```python
from build123d import *

# Parameters (mm, degrees)
SKETCH1_W                                      = 120
SKETCH1_H                                      = 120
BOSS_EXTRUDE1_DEPTH                            = 3
SKETCH2_R                                      = 16
BOSS_EXTRUDE2_DEPTH                            = 8
BOSS_EXTRUDE2_DIRECTION_2_REACH                = 122.252
SKETCH3_R                                      = 13.75
CUT_EXTRUDE1_DEPTH                             = 122.407232036
CHAMFER1_SIZE                                  = 5
CSK_FOR_5_FLAT_HEAD_MACHINE_SCREW2_D           = 3.9116
CSK_FOR_5_FLAT_HEAD_MACHINE_SCREW2_DEPTH       = 10.1
CSK_FOR_5_FLAT_HEAD_MACHINE_SCREW2_CSINK_D     = 6.4008
CSK_FOR_5_FLAT_HEAD_MACHINE_SCREW2_CSINK_ANGLE = 82
CSK_FOR_5_FLAT_HEAD_MACHINE_SCREW2_TIP         = 1.175163199


with BuildPart() as part:
    # Sketch1 → Boss-Extrude1 (new body)
    with BuildSketch(Plane(origin=(0, 0, 0), x_dir=(1, 0, 0), z_dir=(0, 1, 0))):
        with Locations((0, -44)):
            Rectangle(SKETCH1_W, SKETCH1_H)
    extrude(amount=-BOSS_EXTRUDE1_DEPTH)

    # Sketch2 → Boss-Extrude2 (add)
    with BuildSketch(Plane(origin=(0, 1.389185421, -0.121537976), x_dir=(-1, 0, 0), z_dir=(0, 0.9961946980917455, -0.08715574274765836))):
        with Locations(Location((0, 0, 0), (0, 0, 90))):
            Circle(SKETCH2_R)
    extrude(amount=BOSS_EXTRUDE2_DEPTH)

    # Boss-Extrude2 direction 2: up to this face of the body (flat: up to its plane)
    boss_extrude2_direction_2_end = Plane(part.part.faces().sort_by_distance((0, 0, 44))[0])
    # Sketch2 → Boss-Extrude2 direction 2 (add, up to the picked face)
    with BuildSketch(Plane(origin=(0, 1.389185421, -0.121537976), x_dir=(-1, 0, 0), z_dir=(0, 0.9961946980917455, -0.08715574274765836)), mode=Mode.PRIVATE) as boss_extrude2_direction_2_sk1:
        with Locations(Location((0, 0, 0), (0, 0, 90))):
            Circle(SKETCH2_R)
    boss_extrude2_direction_2_tool1 = split(extrude(boss_extrude2_direction_2_sk1.sketch, amount=-BOSS_EXTRUDE2_DIRECTION_2_REACH, mode=Mode.PRIVATE), bisect_by=boss_extrude2_direction_2_end, keep=Keep.BOTH, mode=Mode.PRIVATE)
    add(boss_extrude2_direction_2_tool1.solids().sort_by(Axis((0, 1.389185, -0.121538), (0, -0.9961946980917455, 0.08715574274765836)))[0])

    # Sketch3 → Cut-Extrude1 (cut, through all)
    with BuildSketch(Plane(origin=(0, 9.358743006, -0.818783918), x_dir=(1, 0, 0), z_dir=(0, 0.9961946980917457, -0.08715574274765836))):
        with Locations(Location((0, 0, 0), (0, 0, 270))):
            Circle(SKETCH3_R)
    extrude(amount=-CUT_EXTRUDE1_DEPTH, mode=Mode.SUBTRACT)

    # Chamfer1
    # the kernel refuses this chamfer: 5 mm, written as the material it takes off along each edge
    with BuildSketch(Plane(origin=(60, 0, -28.85841494), x_dir=(-0.9996219169112968, 0.027495876610586372, 0), z_dir=(0, 0, 1)), Plane(origin=(72.85841494, 0, 104), x_dir=(0, 0.027495876610586334, -0.9996219169112968), z_dir=(-1, 0, 0)), Plane(origin=(-60, 0, 116.85841494), x_dir=(0.9996219169112968, 0.027495876610586372, 0), z_dir=(0, 0, -1))) as chamfer1_piece_1:
        Polygon((CHAMFER1_SIZE * 0.999621916911, CHAMFER1_SIZE * 0.0274958766106), (-CHAMFER1_SIZE * 0.0274958766106, CHAMFER1_SIZE * 0.999621916911), (0, 0), align=None)
    extrude(amount=145.71682988, mode=Mode.SUBTRACT)

    # CSK for #5 Flat Head Machine Screw2
    with Locations(Plane(origin=(0, 4.243645214, -16.432388249), x_dir=(0, -0.996194698092, 0.087155742748), z_dir=(0, -0.087155742748, -0.996194698092))):
        with Locations((0, 0)):
            CounterSinkHole(CSK_FOR_5_FLAT_HEAD_MACHINE_SCREW2_D / 2, CSK_FOR_5_FLAT_HEAD_MACHINE_SCREW2_CSINK_D / 2, depth=CSK_FOR_5_FLAT_HEAD_MACHINE_SCREW2_DEPTH, counter_sink_angle=CSK_FOR_5_FLAT_HEAD_MACHINE_SCREW2_CSINK_ANGLE)
            with Locations((0, 0, -(CSK_FOR_5_FLAT_HEAD_MACHINE_SCREW2_DEPTH + CSK_FOR_5_FLAT_HEAD_MACHINE_SCREW2_TIP / 2))):  # 118° drill point
                Cone(0, CSK_FOR_5_FLAT_HEAD_MACHINE_SCREW2_D / 2, CSK_FOR_5_FLAT_HEAD_MACHINE_SCREW2_TIP, mode=Mode.SUBTRACT)


solid = part.part
```
The listing builds one solid part. Answer for the finished solid, in the listing's coordinates (mm). Round coordinates to 2 decimals unless told otherwise and drop trailing zeros. Write each loop counter-clockwise with the first axis right and the second up, starting at its lowest first coordinate (ties: lowest second). Pieces come first, ordered by that corner, then holes. Notation, with made-up numbers: (85.25, 21.25) -> (90.25, 21.25) arc R19 ccw to (90.25, 47.25) -> close; hole circle Ø10 at (-10, -3). An arc over 180 degrees is marked (long way). Answer as a JSON object with one key per item and string values. Group by question number.
Q1. Each of these flat-tipped pins is pushed along its axis until it touches: pin 1 Ø1.5 at (x, y) = (27, -1.5) entering from -Z; pin 2 Ø8 at (x, z) = (17.5, 78) entering from +Y. Where does it stop, or does it pass through?
Q2. Section A-A (x = 33) is taken. Write down the section's boundary in (y, z), plus the area to 4 significant figures.
Q3. Determine the mould class of faces 1 (the face through (0.75, 6.21, -14.68)), 2 (the face through (-1, -3, 42)), 3 (the face through (56, -1, 42)), 4 (the face through (-5.266, 3.782, 12.419)) for opening direction X: pulls with the +X half, pulls with the -X half, needs draft (parallel to the pull), parting line crosses it, or undercut.
Q4. Straight lines are drawn through the part: line 1 along Y through (x, z) = (49, 24.5); line 2 along X through (y, z) = (3.75, 2.5); line 3 along Z through (x, y) = (-11, 7.5). For each, find the intervals that lie inside material, in ascending order.
Q5. Section B-B (z = 74.5) is taken. Write down the section's boundary in (x, y), plus the area to 3 significant figures.
Check values:
{
 "1": {"pin 1": "z = -16", "pin 2": "y = 0"},
 "2": {"outline": "(-3, -16) -> (0, -16) -> (0, 99) -> (-3, 102) -> close", "area": "349.5 mm^2"},
 "3": {"face 1": "undercut", "face 2": "needs draft", "face 3": "pulls with the +X half", "face 4": "undercut"},
 "4": {"line 1": "-3 to 0", "line 2": "-15.75 to -13.46, 13.46 to 15.75", "line 3": "-12.32 to -8.94, 7.63 to 11.01"},
 "5": {"outline": "(-58, -3) -> (58, -3) -> (55, 0) -> (-55, 0) -> close", "area": "339 mm^2"}
}
